Read the model definition and answer for the solid it produces. Units are mm, in the model's axes. A direction names the side the tool comes from. Coordinates: 2 decimals unless noted, no trailing zeros. Order: outer loops, then holes, each group sorted by start corner. A loop starts at its lowest first (then second) coordinate and runs counter-clockwise, first axis right, second up. Notation, with made-up numbers: (76.5, -18.5) -> (98.5, -18.5) arc R32 cw to (98.5, 8.5) -> close; hole circle Ø3 at (26, -9.5). An arc over 180 degrees is marked (long way). Use CSV: the item, a comma, the result in double quotes.
```python
from build123d import *

# Parameters (mm, degrees)
EXTRUDE_1_DEPTH              = 4
FILLET_1_R                   = 10
FILLET_2_R                   = 1
SKETCH_2_W                   = 21
SKETCH_2_H                   = 6
EXTRUDE_2_DEPTH              = 2
SKETCH_3_R                   = 4
EXTRUDE_3_DEPTH              = 6
HOLE_WIZARD_M2_1_D           = 2.6
HOLE_WIZARD_M2_1_CBORE_D     = 6.2
HOLE_WIZARD_M2_1_CBORE_DEPTH = 2
CHAMFER_1_SIZE               = 3
EXTRUDE_4_DEPTH              = 6
CUT_EXTRUDE_2_DEPTH          = 0.75
HOLE_WIZARD_M2_2_D           = 8
HOLE_WIZARD_M2_2_CBORE_D     = 16
HOLE_WIZARD_M2_2_CBORE_DEPTH = 2
SKETCH_9_R                   = 1
CUT_EXTRUDE_1_DEPTH          = 2
PATTERN_CIRCULAR_1_COUNT     = 8


with BuildPart() as part:
    # ｽｹｯﾁ1 → ﾎﾞｽ - 押し出し1 (new body)
    with BuildSketch(Plane(origin=(0, 0, 0), x_dir=(1, 0, 0), z_dir=(0, 1, 0))):
        with BuildLine():
            Line((21.04554885, 3), (19, 3))
            Line((19, 3), (-10.5, 3))
            Line((-10.5, 3), (-10.5, -3))
            Line((-10.5, -3), (32, -3))
            ThreePointArc((32, -3), (25.755002002, -1.401754251), (21.04554885, 3))
        make_face()
        with BuildLine():
            Line((19.049468925, 8.866975344), (19, 8.862647374))
            Line((19, 8.862647374), (19, 3))
            Line((19, 3), (21.04554885, 3))
            ThreePointArc((21.04554885, 3), (19.692790986, 5.812804485), (19.049468925, 8.866975344))
        make_face()
        with BuildLine():
            Line((20.543760972, 8.997708958), (19.049468925, 8.866975344))
            ThreePointArc((19.049468925, 8.866975344), (19.692790986, 5.812804485), (21.04554885, 3))
            Line((21.04554885, 3), (22.875856205, 3))
            ThreePointArc((22.875856205, 3), (21.281736732, 5.832406867), (20.543760972, 8.997708958))
        make_face()
        with BuildLine():
            Line((32, 10), (20.543760972, 8.997708958))
            ThreePointArc((20.543760972, 8.997708958), (21.281736732, 5.832406867), (22.875856205, 3))
            Line((22.875856205, 3), (32, 3))
            Line((32, 3), (32, -1.5))
            ThreePointArc((32, -1.5), (39.000756434, 0.876436587), (43.108147002, 7.023580981))
            Line((43.108147002, 7.023580981), (32, 10))
        make_face()
        with BuildLine():
            ThreePointArc((43.5, 10), (31.498377045, 21.489054548), (20.543760972, 8.997708958))
            Line((20.543760972, 8.997708958), (32, 10))
            Line((32, 10), (43.108147002, 7.023580981))
            ThreePointArc((43.108147002, 7.023580981), (43.401615906, 8.498948789), (43.5, 10))
        make_face()
        with BuildLine():
            Line((32, 3), (22.875856205, 3))
            ThreePointArc((22.875856205, 3), (26.913252513, -0.313825672), (32, -1.5))
            Line((32, -1.5), (32, 3))
        make_face()
        with BuildLine():
            Line((22.875856205, 3), (21.04554885, 3))
            ThreePointArc((21.04554885, 3), (25.755002002, -1.401754251), (32, -3))
            Line((32, -3), (32, -1.5))
            ThreePointArc((32, -1.5), (26.913252513, -0.313825672), (22.875856205, 3))
        make_face()
        with BuildLine():
            ThreePointArc((32, -3), (39.913898577, -0.313593424), (44.557035742, 6.635352414))
            Line((44.557035742, 6.635352414), (43.108147002, 7.023580981))
            ThreePointArc((43.108147002, 7.023580981), (39.000756434, 0.876436587), (32, -1.5))
            Line((32, -1.5), (32, -3))
        make_face()
    extrude(amount=EXTRUDE_1_DEPTH)

    # ﾌｨﾚｯﾄ1
    # the kernel refuses this fillet: 10 mm, written as the material it adds along each edge
    with BuildSketch(Plane(origin=(19, 0, -3), x_dir=(-1, 0, 0), z_dir=(0, 1, 0))) as fillet_1_piece_1:
        with BuildLine():
            CenterArc((9.103972388, -10), FILLET_1_R, 90, 65.560304835)
            Line((0, -5.862647374), (-0.182079448, -5.779900322))
            ThreePointArc((-0.182079448, -5.779900322), (-0.2, -2.931323687), (-0.2, 0))
            Line((-0.2, 0), (0, 0.2))
            Line((0, 0.2), (9.103972388, 0.2))
            Line((9.103972388, 0.2), (9.103972388, 0))
        make_face()
    extrude(amount=4)

    # ﾌｨﾚｯﾄ2
    fillet_2_edges = [part.edges().sort_by_distance(p)[0] for p in [
        (44.557035742, 2, -6.635352414),
        (19, 2, -8.862647374),
    ]]
    fillet(fillet_2_edges, radius=FILLET_2_R)

    # ｽｹｯﾁ2 → ﾎﾞｽ - 押し出し2 (add)
    with BuildSketch(Plane(origin=(0, 4, 0), x_dir=(1, 0, 0), z_dir=(0, 1, 0))):
        Rectangle(SKETCH_2_W, SKETCH_2_H)
    extrude(amount=EXTRUDE_2_DEPTH)

    # ｽｹｯﾁ3 → ﾎﾞｽ - 押し出し3 (add)
    with BuildSketch(Plane(origin=(0, 6, 0), x_dir=(1, 0, 0), z_dir=(0, 1, 0))):
        Circle(SKETCH_3_R)
    extrude(amount=-EXTRUDE_3_DEPTH)

    # M2 丸平ねじ用座ぐり穴1 (through all)
    with Locations(Plane(origin=(0, 0, 0), x_dir=(-1, 0, 0), z_dir=(0, -1, 0))):
        with Locations((0, 0)):
            CounterBoreHole(HOLE_WIZARD_M2_1_D / 2, HOLE_WIZARD_M2_1_CBORE_D / 2, HOLE_WIZARD_M2_1_CBORE_DEPTH)

    # 面取り1
    chamfer_1_edges = [part.edges().sort_by_distance(p)[0] for p in [
        (-10.5, 0, 0),
    ]]
    chamfer(chamfer_1_edges, length=CHAMFER_1_SIZE)

    # ｽｹｯﾁ6 → ﾎﾞｽ - 押し出し4 (add)
    with BuildSketch(Plane.XY.offset(3)):
        Polygon((3, 6), (4.5, 9.5), (7, 9.5), (7.9, 6), align=None)
    extrude_4 = extrude(amount=-EXTRUDE_4_DEPTH)

    # ｽｹｯﾁ10 → ｶｯﾄ - 押し出し2 (cut, symmetric)
    with BuildSketch(Plane.XY):
        Polygon((5, 9.5), (4.5, 9.5), (3, 6), (3.5, 6), align=None)
        Polygon((6.5, 9.5), (7, 9.5), (7.9, 6), (7.4, 6), align=None)
    cut_extrude_2 = extrude(amount=CUT_EXTRUDE_2_DEPTH, both=True, mode=Mode.SUBTRACT)

    # ﾐﾗｰ1: ﾎﾞｽ - 押し出し4, ｶｯﾄ - 押し出し2 across plane
    add(extrude_4.mirror(Plane(origin=(0, 0, 0), x_dir=(0, 0, 1), z_dir=(1, 0, 0))))
    add(cut_extrude_2.mirror(Plane(origin=(0, 0, 0), x_dir=(0, 0, 1), z_dir=(1, 0, 0))), mode=Mode.SUBTRACT)

    # M2 丸平ねじ用座ぐり穴2 (through all)
    with Locations(Plane(origin=(0, 4, 0), x_dir=(1, 0, 0), z_dir=(0, 1, 0))):
        with Locations((32, 10)):
            CounterBoreHole(HOLE_WIZARD_M2_2_D / 2, HOLE_WIZARD_M2_2_CBORE_D / 2, HOLE_WIZARD_M2_2_CBORE_DEPTH)

    # ｽｹｯﾁ9 → ｶｯﾄ - 押し出し1 (cut)
    with BuildSketch(Plane(origin=(0, 2, 0), x_dir=(1, 0, 0), z_dir=(0, 1, 0))):
        with Locations(Location((29.703899406, 15.543277195, 0), (0, 0, 270))):
            Circle(SKETCH_9_R)
    cut_extrude_1 = extrude(amount=-CUT_EXTRUDE_1_DEPTH, mode=Mode.SUBTRACT)

    # 円形ﾊﾟﾀｰﾝ1: ｶｯﾄ - 押し出し1 ×8 about axis
    pattern_circular_1_axis = Axis((32, 0, -10), (0, 1, 0))
    for i in range(1, PATTERN_CIRCULAR_1_COUNT):
        add(cut_extrude_1.rotate(pattern_circular_1_axis, i * 360 / PATTERN_CIRCULAR_1_COUNT), mode=Mode.SUBTRACT)


solid = part.part
```
Item 1: A tool of negligible diameter and unlimited length cuts with its end or side. For faces 4 (the cylindrical face through (39.385, 1.972, 0.698)), 5 (the flat face through (7.2, 7.8, -0.75)), 6 (the flat face through (-3.92, 7.76, 0.75)), from which of +Z, -Z, +X, -X, +Y, -Y can it reach the whole face along a straight path? Write none if from no direction.
Return value:
face 4,"+Z, +X, +Y, -Y"
face 5,"+X, +Y"
face 6,"+Y"
Item 2: Find section D-D, the plane x = -6. Give the vertices of the cut face in (y, z), then the cut area to 3 significant figures.
Return value:
outline,"(0, -3) -> (9.5, -3) -> (9.5, 3) -> (0, 3) -> close"
area,"57.0 mm^2"
Item 3: Straight lines are drawn through the part: line 1 along Z through (x, y) = (32, 0.7); line 2 along Y through (x, z) = (0.5, 2); line 3 along Y through (x, z) = (36, -7). For each, find the intervals that lie inside material, in ascending order.
Return value:
line 1,"z = -21.5 to -14, -6 to 3"
line 2,"y = 2 to 6"
line 3,"y = 0 to 2"
Item 4: Find section C-C, the plane z = 0. Give the vertices of the cut face in (x, y).
Return value:
outline,"(-10.5, 3) -> (-7.5, 0) -> (-3.1, 0) -> (-3.1, 2) -> (-1.3, 2) -> (-1.3, 6) -> (-3.5, 6) -> (-5, 9.5) -> (-6.5, 9.5) -> (-7.4, 6) -> (-10.5, 6) -> close; (1.3, 2) -> (3.1, 2) -> (3.1, 0) -> (40.31, 0) -> (40.31, 4) -> (10.5, 4) -> (10.5, 6) -> (7.4, 6) -> (6.5, 9.5) -> (5, 9.5) -> (3.5, 6) -> (1.3, 6) -> close"
Item 5: The mould has two halves that part along Z. Classify faces 1 (the cylindrical face through (25.613, 1.014, -11.759)), 2 (the flat face through (-6, 5, 3)), 3 (the flat face through (-6, 9.5, 0)): +Z half, -Z half, draft (parallel to the pull), parting line (faces both ways), or undercut.
Return value:
face 1,"undercut"
face 2,"+Z half"
face 3,"draft"
Item 6: Find section B-B, the plane y = 5. Give the vertices of the cut face in (x, z), then the cut area to 3 significant figures.
Return value:
outline,"(-10.5, -3) -> (-2.65, -3) arc R4 ccw to (2.65, -3) -> (10.5, -3) -> (10.5, 3) -> (2.65, 3) arc R4 ccw to (-2.65, 3) -> (-10.5, 3) -> close; hole circle Ø2.6 at (0, 0)"
area,"128 mm^2"
Item 7: Each of these flat-tipped pins is pushed along its axis until it touches: P1, Ø1.6, axis at x = 3.5, y = 7.5, coming from the +Z side; P2, Ø4, axis at x = 13.5, y = 5.5, coming from the -Z side; P3, Ø1.1, axis at x = -7.5, y = 8, coming from the -Z side; P4, Ø1.6, axis at x = 0, z = 0, coming from the -Y side. Where does it stop, or does it pass through?
Return value:
P1,"stops at z = 3"
P2,"stops at z = -4.3"
P3,"stops at z = -3"
P4,"passes through"
Item 8: Find section A-A, the plane y = 7.75. Give the vertices of the cut face in (x, z), then the cut area to 3 significant figures.
Return value:
outline,"(-7.45, -3) -> (-3.75, -3) -> (-3.75, -0.75) -> (-4.25, -0.75) -> (-4.25, 0.75) -> (-3.75, 0.75) -> (-3.75, 3) -> (-7.45, 3) -> (-7.45, 0.75) -> (-6.95, 0.75) -> (-6.95, -0.75) -> (-7.45, -0.75) -> close; (3.75, -3) -> (7.45, -3) -> (7.45, -0.75) -> (6.95, -0.75) -> (6.95, 0.75) -> (7.45, 0.75) -> (7.45, 3) -> (3.75, 3) -> (3.75, 0.75) -> (4.25, 0.75) -> (4.25, -0.75) -> (3.75, -0.75) -> close"
area,"41.4 mm^2"
